The listing builds one solid part. Answer for the finished solid, in the listing's coordinates (mm). Coordinates: 2 decimals unless noted, no trailing zeros. Loops run counter-clockwise (first coordinate to the right, second up) from the corner with the lowest first, then second, coordinate; pieces in that order, holes last. Notation, with made-up numbers: (-37.75, -38) -> (17.25, -38) arc R15 ccw to (17.25, -13) -> close; hole circle Ø10 at (17, 65.25). An arc over 180 degrees is marked (long way). Answer in a Markdown table with one row per item.
Autodesk Inventor part; units mm, degrees
ref_plane "YZ Plane" through (0, 0, 0) normal (1, 0, 0) x (0, 1, 0)
ref_plane "XZ Plane" through (0, 0, 0) normal (0, 1, 0) x (-1, 0, 0)
ref_plane "XY Plane" through (0, 0, 0) normal (0, 0, 1) x (1, 0, 0)
sketch "Sketch1" plane through (0, 0, 0) normal (1, 0, 0) x (0, 1, 0)
  line L0 (0, 0) -> (-50.8, 0)
  line L1 (-50.8, 0) -> (-50.8, -3.175)
  line L2 (-50.8, -3.175) -> (0, -3.175)
  line L3 (0, -3.175) -> (0, 0)
  line L4 (0, 0) -> (-3.175, 0)
  line L5 (-3.175, 0) -> (-3.175, -50.8)
  line L6 (-3.175, -50.8) -> (0, -50.8)
  line L7 (0, -50.8) -> (0, 0)
  dimension "d0" = 50.8
  dimension "d1" = 3.175
  dimension "d2" = 3.175
  dimension "d3" = 50.8
extrude "Extrusion1" add sketch "Sketch1" along normal blind 552.45
sketch "Sketch2" plane through (0, 0, 0) normal (0, 1, 0) x (1, 0, 0)
  line L0 (0, 50.8) -> (0, 0)
  line L1 (0, 0) -> (552.45, 0)
  line L2 (552.45, 50.8) -> (552.45, 0)
  line L3 (0, 50.8) -> (552.45, 50.8)
  point P0 (12.7, 12.7)
  point P1 (12.7, 38.1)
  point P2 (539.75, 12.7)
  point P3 (539.75, 38.1)
  dimension "d6" = 12.7
  dimension "d7" = 12.7
  dimension "d8" = 12.7
  dimension "d9" = 12.7
  dimension "d10" = 12.7
  dimension "d11" = 12.7
  dimension "d12" = 12.7
  dimension "d13" = 12.7
hole "Hole1" at (12.7, 0, -12.7) at (12.7, 0, -38.1) at (539.75, 0, -12.7) at (539.75, 0, -38.1) direction (0, -1, 0) diameter 6.35 end through all
properties part number "2x2 angle support"
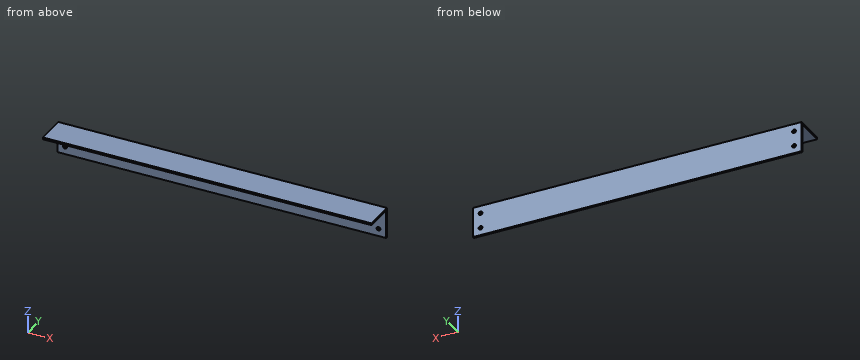
Item 1: Flat-ended cylindrical pins translate along their axes: pin 1 Ø5.5 at (x, z) = (539.75, -38.1) entering from -Y; pin 2 Ø3 at (x, y) = (67, -26.5) entering from -Z (3 decimals); pin 3 Ø7.5 at (x, z) = (12.7, -12.7) entering from -Y (3 decimals). Find the tip coordinate at first contact, or state that the pin passes through.
Findings below:
| item | result |
|---|---|
| pin 1 | passes through |
| pin 2 | stops at z = -3.175 |
| pin 3 | stops at y = -3.175 |
Item 2: A cutting plane is placed at B-B, the plane z = -25.5. Determine the outline of the cut face in (x, y) (3 decimals).
Findings below:
| item | result |
|---|---|
| outline | (0, -3.175) -> (552.45, -3.175) -> (552.45, 0) -> (0, 0) -> close |
Item 3: A cutting plane is placed at A-A, the plane x = 179. Determine the outline of the cut face in (y, z) (3 decimals), plus the area to 4 significant figures.
Findings below:
| item | result |
|---|---|
| outline | (-50.8, -3.175) -> (-3.175, -3.175) -> (-3.175, -50.8) -> (0, -50.8) -> (0, 0) -> (-50.8, 0) -> close |
| area | 312.5 mm2 |
Item 4: Find the intervals of material crossed by probe 1 along Z at (x, y) = (12, -1); probe 2 along Z at (x, y) = (539.75, -2.05) (3 decimals); probe 3 along X at (y, z) = (-1.2, -38.1) (3 decimals), in increasing order.
Findings below:
| item | result |
|---|---|
| probe 1 | z = -50.8 to -41.2, -35 to -15.8, -9.6 to 0 |
| probe 2 | z = -50.8 to -41.275, -34.925 to -15.875, -9.525 to 0 |
| probe 3 | x = 0 to 9.525, 15.875 to 536.575, 542.925 to 552.45 |
